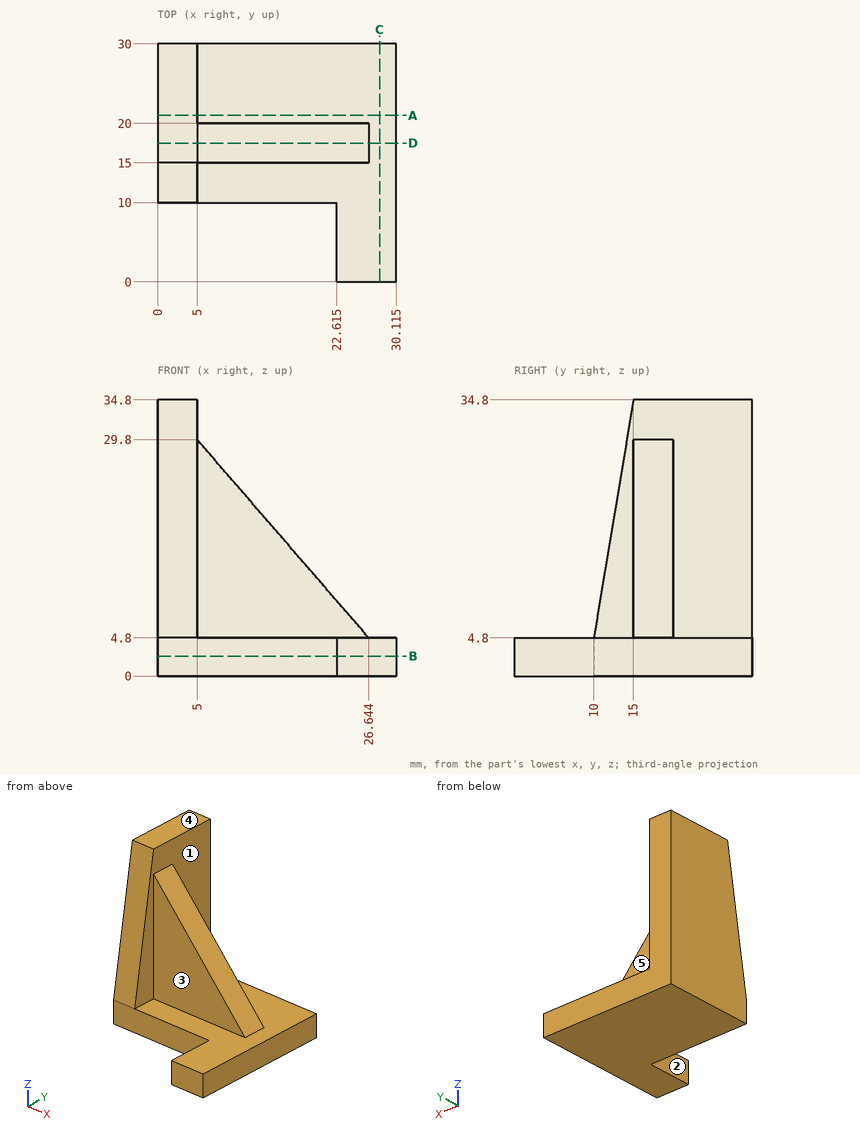
Here's the drawing with two shaded views (mm, measured from the low corner). I have some questions. A direction names the side the tool comes from. Coordinates: 2 decimals unless noted, no trailing zeros. Write each loop counter-clockwise with the first axis right and the second up, starting at its lowest first coordinate (ties: lowest second). Pieces come first, ordered by that corner, then holes. Notation, with made-up numbers: M 30.25,80.5 L 63.25,80.5 A12 cw 63.25,97.5 Z; hole C 87,4.5 d2. An arc over 180 degrees is marked long. Write item = value, one per line. Start each with the question number.
Q1. If we section it at D-D, the plane y = 17.5: Write out the boundary of the cut face in (x, z) (1 decimal), then the cut area to 3 significant figures.
Q2. I'm going to push flat-ended pins straight in: pin 1 (2.5 mm diameter, centred on x = 7.5, z = 2.5, fed in from -Y); pin 2 (6 mm diameter, centred on y = 20, z = 16, fed in from -X); pin 3 (1 mm diameter, centred on y = 25.5, z = 10.5, fed in from +X); pin 4 (6.5 mm diameter, centred on x = 15.5, z = 11.5, fed in from -Y). Where does each tip first touch, or does it pass through?
Q3. If we section it at A-A, the plane y = 21: Write out the boundary of the cut face in (x, z) (1 decimal).
Q4. If we section it at C-C, the plane x = 28: Write out the boundary of the cut face in (y, z).
Q5. If I drill on L1, parallel to Z at x = 22, y = 14.5; L2, parallel to Y at x = 13, z = 18; L3, parallel to X at y = 8.5, z = 2 (1 decimal), over which ranges is the centre line in solid material (lowest first)? Write a range as [from, to].
Q6. On a 3-axis mill with a long thin cutter (end or side, diameter ignored), from which of +Z, -Z, +X, -X, +Y, -Y can I reach the whole of each face in a straight line? I mean the marked faces 1, 2, 3, 4 and 5. Say none if no direction works.
Q7. If we section it at B-B, the plane z = 2.5: Write out the boundary of the cut face in (x, y) (1 decimal).
Check sheet entries:
q1.outline = M 0,0 L 30.1,0 L 30.1,4.8 L 26.6,4.8 L 5,29.8 L 5,34.8 L 0,34.8 Z
q1.area = 565 mm²
q2.pin_1 = 10
q2.pin_2 = 0
q2.pin_3 = 5
q2.pin_4 = 15
q3.outline = M 0,0 L 30.1,0 L 30.1,4.8 L 5,4.8 L 5,34.8 L 0,34.8 Z
q4.outline = M 0,0 L 30,0 L 30,4.8 L 0,4.8 Z
q5.L1 = [0, 4.8]
q5.L2 = [15, 20]
q5.L3 = [22.6, 30.1]
q6.face_1 = +Z, +X
q6.face_2 = +Z, -Z, -X, -Y
q6.face_3 = +Z, +X, -Y
q6.face_4 = +Z, +X, -X, +Y, -Y
q6.face_5 = +Z, +X, +Y
q7.outline = M 0,10 L 22.6,10 L 22.6,0 L 30.1,0 L 30.1,30 L 0,30 Z
